Build history of the part. All positions in model axes, mm. Give positions to 0.01 mm unless a question says otherwise; leave off trailing zeros. Write each loop counter-clockwise with the first axis right and the second up, starting at its lowest first coordinate (ties: lowest second). Pieces come first, ordered by that corner, then holes. Notation, with made-up numbers: (-29.5, 28) -> (-10.5, 28) arc R35 ccw to (-10.5, 67) -> close; hole circle Ø6 at (88.5, 24). An arc over 180 degrees is marked (long way). Write item = value, one per line. Start each with the question number.
Q1. Wall check: line 1 (X direction, y = 104.5, z = 4.75); line 2 (X direction, y = 103, z = 4.5); line 3 (Y direction, x = 16.5, z = 4.75). Give the ranges that are in metal, low to high.
Q2. Saw through at A-A, the plane z = 2. List the corners of the cut face in (x, y), then the cut area to 3 significant figures.
Q3. Saw through at C-C, the plane y = 96. List the corners of the cut face in (x, z), then the cut area to 3 significant figures.
Q4. Saw through at B-B, the plane x = 30. List the corners of the cut face in (y, z), then the cut area to 3 significant figures.
Autodesk Inventor part; units mm, degrees
ref_plane "YZ Plane" through (0, 0, 0) normal (1, 0, 0) x (0, 1, 0)
ref_plane "XZ Plane" through (0, 0, 0) normal (0, 1, 0) x (-1, 0, 0)
ref_plane "XY Plane" through (0, 0, 0) normal (0, 0, 1) x (1, 0, 0)
sketch "Sketch1" plane through (0, 0, 0) normal (0, 0, 1) x (1, 0, 0)
  line L0 (-10.6635, 0) -> (40.1365, 0)
  line L1 (40.1365, 0) -> (40.1365, 127)
  line L2 (14.7365, 127) -> (-10.6635, 127)
  line L3 (-10.6635, 127) -> (-10.6635, 0)
  line L4 (40.1365, 0) -> (40.1365, 25.4)
  arc A0 (40.1365, 25.4) -> (14.7365, 127) centre (-175.7635, 25.4) ccw
  point P0 (0, 0)
  dimension "d0" = 50.8
  dimension "d1" = 127
  dimension "d2" = 25.4
extrude "Extrusion1" add sketch "Sketch1" along normal blind 6.35
fillet "Fillet1" radius 12.7 1 edges at (40.1365, 0, 3.175)
properties part number "Zachs wing"
Report:
q1.line_1 = -10.66 to 25.12
q1.line_2 = -10.66 to 25.71
q1.line_3 = 0 to 123.62
q2.outline = (-10.66, 0) -> (27.44, 0) arc R12.7 ccw to (40.14, 12.7) -> (40.14, 25.4) arc R215.9 ccw to (14.74, 127) -> (-10.66, 127) -> close
q2.area = 5,580 mm2
q3.outline = (-10.66, 0) -> (28.27, 0) -> (28.27, 6.35) -> (-10.66, 6.35) -> close
q3.area = 247 mm2
q4.outline = (0.26, 0) -> (90.78, 0) -> (90.78, 6.35) -> (0.26, 6.35) -> close
q4.area = 575 mm2
